Geometry check sheet. Reference: the model listing, model coordinates, mm. Face numbers are marked on the shaded views. Round coordinates to 2 decimals unless told otherwise and drop trailing zeros. Order: outer loops, then holes, each group sorted by start corner. A loop starts at its lowest first (then second) coordinate and runs counter-clockwise, first axis right, second up. Notation, with made-up numbers: (-33.5, -2.5) - (17.5, -2.5) arc R28 cw to (17.5, 36.5) - close; hole circle Ø9 at (9, 63.5). An arc over 180 degrees is marked (long way). One line per question, with ' | ' between items. Start each with the question number.
Q1. Sectioned sample at C-C, the plane y = 0. Enter the section's corners in (x, z).
Q2. Sectioned sample at D-D, the plane y = 7. Enter the section's corners in (x, z), then the cut area to 3 significant figures.
Q3. Sectioned sample at B-B, the plane x = 13.25. Enter the section's corners in (y, z), then the cut area to 3 significant figures.
Q4. Sectioned sample at A-A, the plane y = -17.5. Enter the section's corners in (x, z), then the cut area to 3 significant figures.
Q5. Material ranges on line 1 along X through (y, z) = (-9, 0.3); line 2 along Y through (x, z) = (11, 1.6); line 3 along X through (y, z) = (0.5, 0.4), recorded low to high.
Q6. Mould release check, pull along X, two halves, no side actions. Record for the marked faces 1 and 2: +X half, -X half, draft (parallel to the pull), parting line (faces both ways), or undercut.
Q7. Gauge pin test, flat ends, axial feed: P1, Ø1.3, axis at x = -20.5, z = 1.5, coming from the -Y side; P2, Ø2.5, axis at x = 19.25, y = 0, coming from the +Z side; P3, Ø3.5, axis at x = -19.25, y = 15, coming from the -Z side. Record the tip position at first contact, or that the pin passes through.
Autodesk Inventor part; units mm, degrees
ref_plane "YZ Plane" through (0, 0, 0) normal (1, 0, 0) x (0, 1, 0)
ref_plane "XZ Plane" through (0, 0, 0) normal (0, 1, 0) x (-1, 0, 0)
ref_plane "XY Plane" through (0, 0, 0) normal (0, 0, 1) x (1, 0, 0)
sketch "スケッチ1" plane through (0, 0, 0) normal (0, 0, 1) x (1, 0, 0)
  line L0 (-24.25, -20) -> (24.25, -20) construction
  line L1 (24.25, -20) -> (24.25, 20)
  line L2 (24.25, 20) -> (-24.25, 20)
  line L3 (-24.25, 20) -> (-24.25, -20)
  line L4 (-24.25, -20) -> (24.25, 20) construction
  line L5 (24.25, -20) -> (-24.25, 20) construction
  circle A0 centre (-15.25, -17.5) radius 1.55
  circle A1 centre (20.25, -17.5) radius 1.55
  line L6 (-9.25, -15) -> (14.25, -15) construction
  line L7 (14.25, -15) -> (14.25, -20) construction
  line L8 (14.25, -20) -> (-9.25, -20) construction
  line L9 (-9.25, -20) -> (-9.25, -15) construction
  line L10 (-24.25, -20) -> (-15.25, -22)
  line L11 (-15.25, -22) -> (20.25, -22)
  line L12 (20.25, -22) -> (24.25, -20)
  line L13 (14.3, -14.95) -> (-9.3, -14.95)
  line L14 (-9.3, -14.95) -> (-9.3, -20.05)
  line L15 (-9.3, -20.05) -> (14.3, -20.05)
  line L16 (14.3, -20.05) -> (14.3, -14.95)
  circle A2 centre (-8.25, -14.95) radius 1.05
  circle A3 centre (-8.25, -20.05) radius 1.05
  circle A4 centre (13.25, -14.95) radius 1.05
  circle A5 centre (13.25, -20.05) radius 1.05
  circle A6 centre (-19.25, 15) radius 1.55
  line L17 (-21.8, 5.05) -> (-19.2, 5.05)
  line L18 (-19.2, 5.05) -> (-19.2, -15.05)
  line L19 (-19.2, -15.05) -> (-21.8, -15.05)
  line L20 (-21.8, -15.05) -> (-21.8, 5.05)
  line L21 (-19.25, 5) -> (-21.75, 5) construction
  line L22 (-21.75, 5) -> (-21.75, -15) construction
  line L23 (-21.75, -15) -> (-19.25, -15) construction
  line L24 (-19.25, -15) -> (-19.25, 5) construction
  line L25 (2.5, -14.95) -> (2.5, -20.05) construction
  circle A7 centre (19.25, 0) radius 1.55
  line L26 (-19.25, 15) -> (19.25, 15) construction
  line L27 (19.25, 15) -> (19.25, 0) construction
  circle A8 centre (-21.8, 4) radius 1.05
  circle A9 centre (-19.2, 4) radius 1.05
  circle A10 centre (-21.8, -14) radius 1.05
  circle A11 centre (-19.2, -14) radius 1.05
  point P0 (0, 0)
  point P1 (-9.25, -17.5)
  dimension "d10" = 2.1
  dimension "d26" = 2.1
  dimension "d0" = 5
  dimension "d3" = 3.1
  dimension "d4" = 35.5
  dimension "d5" = 2
  dimension "d7" = 40
  dimension "d8" = 23.5
  dimension "d9" = 0.05
  dimension "d11" = 3.1
  dimension "d12" = 5
  dimension "d13" = 5
  dimension "d14" = 0.05
  dimension "d15" = 17.75
  dimension "d16" = 48.5
  dimension "d17" = 4
  dimension "d18" = 5
  dimension "d19" = 20
  dimension "d20" = 2.5
  dimension "d21" = 2.5
  dimension "d22" = 5
  dimension "d23" = 15
  dimension "d27" = 25
extrude "押し出し1" add sketch "スケッチ1" along normal blind 3
sketch "スケッチ2" plane through (0, 0, 0) normal (0, 0, -1) x (-1, 0, 0)
  line L0 (-14.3, -20.05) -> (-14.3, -14.95)
  line L1 (-12.2, -14.95) -> (7.2, -14.95)
  line L2 (24.25, 20) -> (-24.25, 20)
  line L3 (-24.25, 20) -> (-24.25, -20)
  line L4 (21.8, -15.05) -> (19.2, -15.05)
  line L5 (19.2, -12.95) -> (19.2, 2.95)
  line L6 (19.2, 5.05) -> (21.8, 5.05)
  circle A0 centre (-19.25, 0) radius 1.55
  line L7 (-20.25, 16) -> (16.25, 16)
  line L8 (16.25, 16) -> (16.25, -11)
  line L9 (16.25, -11) -> (-20.25, -11)
  line L10 (-20.25, -11) -> (-20.25, -2.8284)
  line L11 (-20.25, 16) -> (-20.25, 2.8284)
  arc A1 (-20.25, -2.8284) -> (-20.25, 2.8284) centre (-19.25, 0) ccw
  line L12 (19.25, 5.05) -> (19.25, -15.05) construction
  line L13 (19.2, -15.05) -> (21.8, -15.05)
  line L14 (-14.3, -15) -> (9.3, -15) construction
  line L15 (9.3, -20.05) -> (9.3, -14.95)
  point P0 (0, 0)
  dimension "d28" = 3
  dimension "d29" = 4
  dimension "d30" = 4
  dimension "d31" = 0.05
  dimension "d32" = 3
  dimension "d33" = 0.05
  dimension "d34" = 4
extrude "押し出し2" cut sketch "スケッチ2" against normal blind 2 contours L7 L8 L9 L10 A1 L11
fillet "フィレット1" radius 2 6 edges at (20.25, 2.8284, 1) (20.25, -2.8284, 1) (20.25, 16, 1) (-16.25, 16, 1) (-16.25, -11, 1) (20.25, -11, 1)
equation "\"d13\" = d12"
equation "\"d15\" = 0.5 * d4"
equation "\"d18\" = d13"
properties part number "コックピット_サブフレーム_1_5" material "アセタール樹脂、黒"
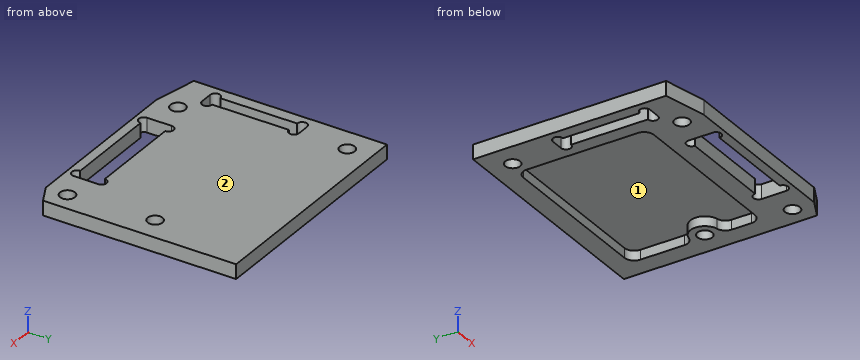
Determined:
1) outline: (-24.25, 0) - (-21.8, 0) - (-21.8, 3) - (-24.25, 3) - close; (-19.2, 0) - (-16.25, 0) - (-16.25, 2) - (16.25, 2) - (16.25, 0) - (17.7, 0) - (17.7, 3) - (-19.2, 3) - close; (20.8, 0) - (24.25, 0) - (24.25, 3) - (20.8, 3) - close
2) outline: (-24.25, 0) - (-16.25, 0) - (-16.25, 2) - (20.25, 2) - (20.25, 0) - (24.25, 0) - (24.25, 3) - (-24.25, 3) - close | area: 72.5 mm2
3) outline: (-22, 0) - (-21.1, 0) - (-21.1, 3) - (-22, 3) - close; (-13.9, 0) - (-11, 0) - (-11, 2) - (16, 2) - (16, 0) - (20, 0) - (20, 3) - (-13.9, 3) - close | area: 50.4 mm2
4) outline: (-24.25, 0) - (-16.8, 0) - (-16.8, 3) - (-24.25, 3) - close; (-13.7, 0) - (-9.3, 0) - (-9.3, 3) - (-13.7, 3) - close; (14.3, 0) - (18.7, 0) - (18.7, 3) - (14.3, 3) - close; (21.8, 0) - (24.25, 0) - (24.25, 3) - (21.8, 3) - close | area: 56.1 mm2
5) line 1: x = -24.25 to -21.8, -19.2 to -16.25, 20.25 to 24.25 | line 2: y = -22 to -20.05, -14.95 to -11, 16 to 20 | line 3: x = -24.25 to -21.8, -19.2 to -16.25, 16.29 to 17.78, 20.72 to 24.25
6) face 1: undercut | face 2: draft
7) P1: stops at y = -20.98 | P2: passes through | P3: stops at z = 0
